The drawing under review shows one solid part. Ordinate dimensions are in mm from its lowest x, y, z. Round coordinates to 2 decimals unless told otherwise and drop trailing zeros. Write each loop counter-clockwise with the first axis right and the second up, starting at its lowest first coordinate (ties: lowest second). Pieces come first, ordered by that corner, then holes.
Item 1: To check wall thickness, follow L1, parallel to Z at x = 60.5, y = 1.15; L2, parallel to X at y = 0.6, z = 13. State the ranges of each line that lie inside material, in increasing order.
Item 2: Add section A-A (z = 66.5). Give the boundary of the cut face in (x, y), plus the area to 3 significant figures.
Item 3: Clearance check with flat-ended pins moving along their axes: pin 1 Ø4 at (x, z) = (33, 73) entering from -Y; pin 2 Ø2 at (y, z) = (0.5, 35) entering from -X; pin 3 Ø1.6 at (x, y) = (24.5, 1) entering from -Z. State where each tip first meets the part, or that it passes through.
Item 4: Add section B-B (y = 1.3). Give the boundary of the cut face in (x, z), plus the area to 3 significant figures.
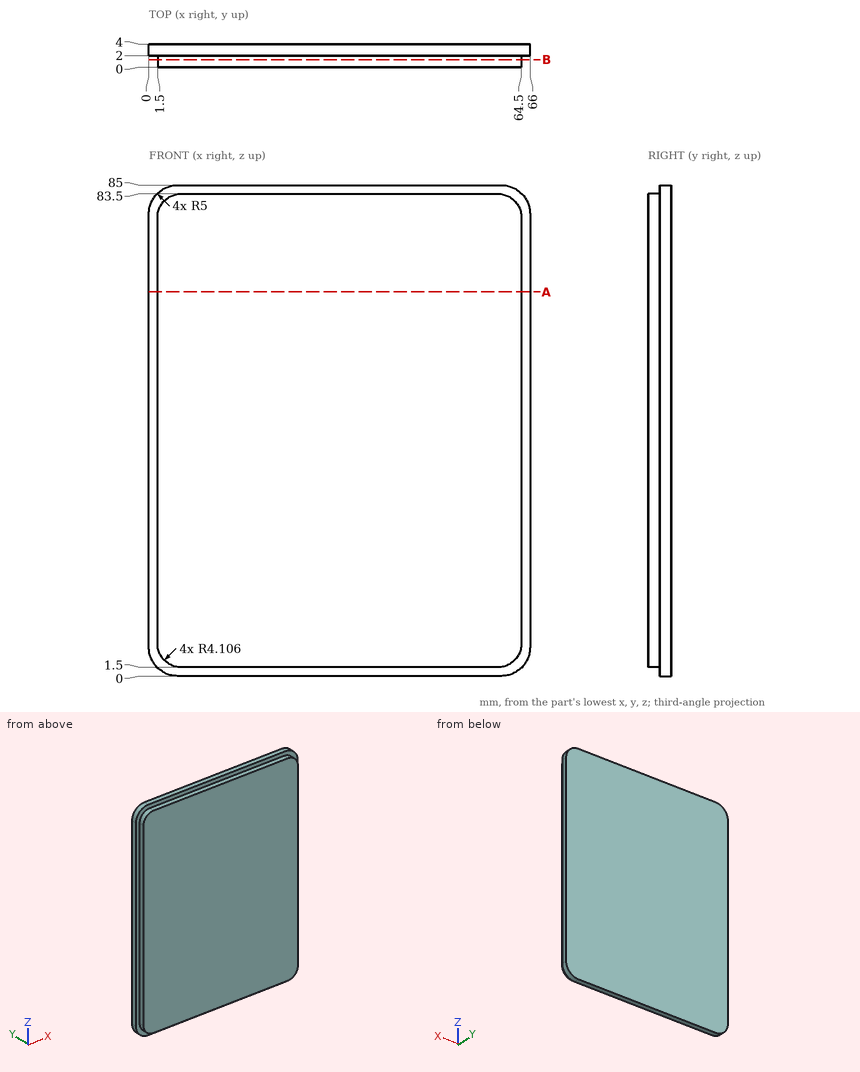
Numbers:
1. L1: z = 1.5 to 83.5
1. L2: x = 1.5 to 64.5
2. outline: (0, 2) - (1.5, 2) - (1.5, 0) - (64.5, 0) - (64.5, 2) - (66, 2) - (66, 4) - (0, 4) - close
2. area: 258 mm2
3. pin 1: stops at y = 0
3. pin 2: stops at x = 1.5
3. pin 3: stops at z = 1.5
4. outline: (1.5, 5.61) arc R4.11 ccw to (5.61, 1.5) - (60.39, 1.5) arc R4.11 ccw to (64.5, 5.61) - (64.5, 79.39) arc R4.11 ccw to (60.39, 83.5) - (5.61, 83.5) arc R4.11 ccw to (1.5, 79.39) - close
4. area: 5,150 mm2
